from build123d import *

# Parameters (mm, degrees)
PAD003_DEPTH = 10
PAD002_DEPTH = 20


with BuildPart() as printbolthead001:
    # Sketch003 → Pad003 (new body)
    with BuildSketch(Plane.XY):
        with BuildLine():
            ThreePointArc((-3.535526, 3.535542), (-1.8e-05, -5), (3.535551, 3.535517))
            Line((2.071068, 5), (3.535551, 3.535517))
            Line((-2.071068, 5), (2.071068, 5))
            Line((-3.535526, 3.535542), (-2.071068, 5))
        make_face()
    extrude(amount=PAD003_DEPTH)


with BuildPart() as printboltslot:
    # Sketch002 → Pad002 (new body)
    with BuildSketch(Plane.XY):
        with BuildLine():
            ThreePointArc((-1.414208, 1.414219), (1e-06, -2), (1.414206, 1.414221))
            Line((0.828427, 2), (1.414206, 1.414221))
            Line((-0.828427, 2), (0.828427, 2))
            Line((-1.414208, 1.414219), (-0.828427, 2))
        make_face()
    extrude(amount=-PAD002_DEPTH)

    # Fusion001: union PrintBoltHead001
    add(printbolthead001.part)


solid = printboltslot.part
Verification items for the finished model (mm, model axes). A direction names the side the tool comes from. Round coordinates to 2 decimals unless told otherwise and drop trailing zeros. Loops run counter-clockwise (first coordinate to the right, second up) from the corner with the lowest first, then second, coordinate; pieces in that order, holes last. Notation, with made-up numbers: (-0.5, -34.75) - (38.5, -34.75) arc R26 cw to (38.5, -12.75) - close; hole circle Ø6 at (17.5, 57). An arc over 180 degrees is marked (long way). Answer in a Markdown table with one row per item. Add a question column.
Q1. Gauge pin test, flat ends, axial feed: pin 1 (2 mm diameter, centred on x = -3.5, y = -2, fed in from -Z); pin 2 (1.8 mm diameter, centred on x = 0, z = -14, fed in from +Y); pin 3 (4 mm diameter, centred on y = 1, z = -13.5, fed in from +X). Record the tip position at first contact, or that the pin passes through.
Q2. Material ranges on line 1 (Z direction, x = -2.75, y = -4); line 2 (Y direction, x = -4.25, z = 6.25); line 3 (X direction, y = -2.5, z = 6.25), recorded low to high.
Q3. Tool access check on faces 1 (the face through (-2.81, 4.26, 4.93)), 2 (the face through (0, 2, -10)), 3 (the face through (2.2, 0.1, 0)). Record the directions out of +Z, -Z, +X, -X, +Y, -Y that give a thin tool (end or side, any length) a straight path to the whole face; none if there is none.
Q4. Section check D-D on y = -3. Enter the section's corners in (x, z), plus the area to 3 significant figures.
Q5. Section check A-A on x = 0. Enter the section's corners in (y, z).
Q6. Section check C-C on z = 2.5. Enter the section's corners in (x, y), plus the area to 3 significant figures.
Found:
| question | item | result |
|---|---|---|
| 1 | pin 1 | stops at z = 0 |
| 1 | pin 2 | stops at y = 2 |
| 1 | pin 3 | stops at x = 2 |
| 2 | line 1 | z = 0 to 10 |
| 2 | line 2 | y = -2.63 to 2.63 |
| 2 | line 3 | x = -4.33 to 4.33 |
| 3 | face 1 | +Z, -Z, -X, +Y |
| 3 | face 2 | -Z, +X, -X, +Y |
| 3 | face 3 | -Z |
| 4 | outline | (-4, 0) - (4, 0) - (4, 10) - (-4, 10) - close |
| 4 | area | 80.0 mm² |
| 5 | outline | (-5, 0) - (-2, 0) - (-2, -20) - (2, -20) - (2, 0) - (5, 0) - (5, 10) - (-5, 10) - close |
| 6 | outline | (-3.54, 3.54) arc R5 ccw (long way) to (3.54, 3.54) - (2.07, 5) - (-2.07, 5) - close |
| 6 | area | 79.6 mm² |
